Part print with two shaded views. Sizes in mm from the minimum x, y, z corner. A direction names the side the tool comes from. Round coordinates to 2 decimals unless told otherwise and drop trailing zeros. Write each loop counter-clockwise with the first axis right and the second up, starting at its lowest first coordinate (ties: lowest second). Pieces come first, ordered by that corner, then holes. Notation, with made-up numbers: (-16.75, 40) - (35.25, 40) arc R26 ccw to (35.25, 79) - close; hole circle Ø2 at (31, 38). An arc over 180 degrees is marked (long way). Answer as a JSON object with one key per item and string values. Group by question number.
Item 1: Flat gauge pins, fed straight in: pin 1 (0.6 mm diameter, centred on x = 4.5, z = 2.5, fed in from +Y); pin 2 (2 mm diameter, centred on x = 3, z = 1.5, fed in from -Y); pin 3 (2 mm diameter, centred on x = 15, z = 3, fed in from +Y). Where does each tip first touch, or does it go through?
Item 2: Two-plate mould, pull along X, no slides. Class the marked faces 4, 5 and 6: +X half, -X half, draft (parallel to the pull), parting line (faces both ways), or undercut.
Item 3: Slice it at C-C, the plane z = 3.1. List the corners of the cut face in (x, y), then the cut area to 3 significant figures.
Item 4: Slice it at B-B, the plane x = 8. List the corners of the cut face in (y, z), then the cut area to 4 significant figures.
Item 5: Probe line 1 (Y direction, x = 8, z = 2.05); line 2 (X direction, y = 6, z = 0.4); line 3 (Y direction, x = 2.5, z = 0.7). List the from-to ranges inside material, lowest first. Write a range as from..to.
Item 6: Slice it at D-D, the plane y = 48.5. List the corners of the cut face in (x, z).
Item 7: Which spindle directions (+Z, -Z, +X, -X, +Y, -Y) get a long thin tool onto all of the face, cutting with end or side? Do the marked faces 1, 2 and 3. Say none if no direction does.
Item 8: Slice it at A-A, the plane y = 40. List the corners of the cut face in (x, z), then the cut area to 3 significant figures.
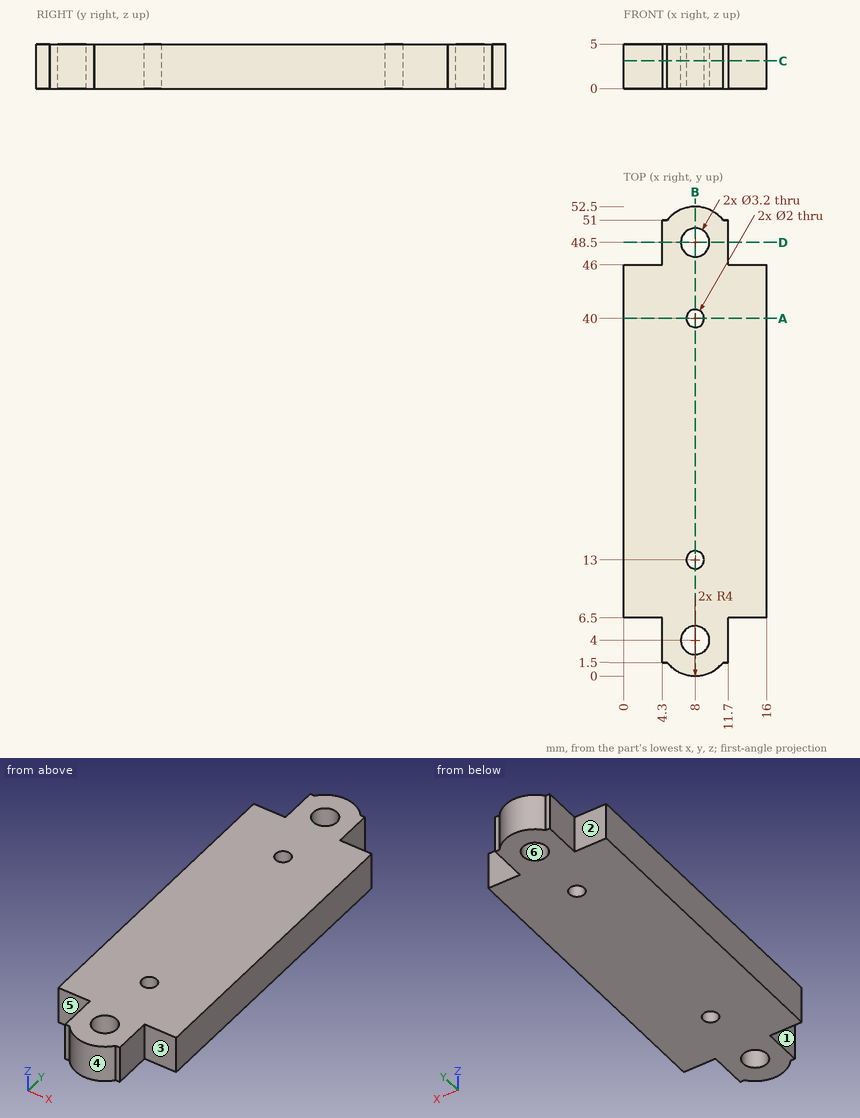
Geometry says:
{
 "1": {"pin 1": "stops at y = 51", "pin 2": "stops at y = 6.5", "pin 3": "stops at y = 46"},
 "2": {"face 4": "parting line", "face 5": "draft", "face 6": "undercut"},
 "3": {"outline": "(0, 6.5) - (4.3, 6.5) - (4.3, 1.5) - (4.88, 1.5) arc R4 ccw to (11.12, 1.5) - (11.7, 1.5) - (11.7, 6.5) - (16, 6.5) - (16, 46) - (11.7, 46) - (11.7, 51) - (11.12, 51) arc R4 ccw to (4.88, 51) - (4.3, 51) - (4.3, 46) - (0, 46) - close; hole circle Ø3.2 at (8, 4); hole circle Ø3.2 at (8, 48.5); hole circle Ø2 at (8, 13); hole circle Ø2 at (8, 40)", "area": "697 mm^2"},
 "4": {"outline": "(0, 0) - (2.4, 0) - (2.4, 5) - (0, 5) - close; (5.6, 0) - (12, 0) - (12, 5) - (5.6, 5) - close; (14, 0) - (39, 0) - (39, 5) - (14, 5) - close; (41, 0) - (46.9, 0) - (46.9, 5) - (41, 5) - close; (50.1, 0) - (52.5, 0) - (52.5, 5) - (50.1, 5) - close", "area": "210.5 mm^2"},
 "5": {"line 1": "y = 0..2.4, 5.6..12, 14..39, 41..46.9, 50.1..52.5", "line 2": "x = 4.3..11.7", "line 3": "y = 6.5..46"},
 "6": {"outline": "(4.3, 0) - (6.4, 0) - (6.4, 5) - (4.3, 5) - close; (9.6, 0) - (11.7, 0) - (11.7, 5) - (9.6, 5) - close"},
 "7": {"face 1": "+Z, -Z, -X, -Y", "face 2": "+Z, -Z, -X, +Y", "face 3": "+Z, -Z, +X, -Y"},
 "8": {"outline": "(0, 0) - (7, 0) - (7, 5) - (0, 5) - close; (9, 0) - (16, 0) - (16, 5) - (9, 5) - close", "area": "70.0 mm^2"}
}
